The model under review builds one solid part; all positions refer to its coordinate system, in mm. A direction names the side the tool comes from. Give positions to 0.01 mm unless a question says otherwise; leave off trailing zeros. Write each loop counter-clockwise with the first axis right and the second up, starting at its lowest first coordinate (ties: lowest second). Pieces come first, ordered by that corner, then holes. Notation, with made-up numbers: (44.25, -10.5) - (67.25, -10.5) arc R28 ccw to (67.25, 7.5) - close; hole circle Ø3 at (35, 31.5). An arc over 180 degrees is marked (long way). One line per question, with ' | ' between items. Start each with the question number.
```python
from build123d import *

# Parameters (mm, degrees)
SKETCH1_W           = 80
SKETCH1_H           = 91
BOSS_EXTRUDE1_DEPTH = 10
SKETCH2_R           = 6.525
CUT_EXTRUDE1_DEPTH  = 76.543960712
SKETCH3_R           = 7.55
CUT_EXTRUDE2_DEPTH  = 1.1
CUT_EXTRUDE3_DEPTH  = 3
CIRPATTERN1_COUNT   = 3
SKETCH5_R           = 2.25
CUT_EXTRUDE4_DEPTH  = 76.543960712
SKETCH6_W           = 15
SKETCH6_H           = 60
CUT_EXTRUDE5_DEPTH  = 3.4
SKETCH7_R           = 1.75
CUT_EXTRUDE6_DEPTH  = 76.169475188


with BuildPart() as part:
    # Sketch1 → Boss-Extrude1 (new body)
    with BuildSketch(Plane.XY):
        with Locations((0, 17.8)):
            Rectangle(SKETCH1_W, SKETCH1_H)
    extrude(amount=BOSS_EXTRUDE1_DEPTH)

    # Sketch2 → Cut-Extrude1 (cut, through all)
    with BuildSketch(Plane.XY.offset(10)):
        Circle(SKETCH2_R)
    extrude(amount=-CUT_EXTRUDE1_DEPTH, mode=Mode.SUBTRACT)

    # Sketch3 → Cut-Extrude2 (cut)
    with BuildSketch(Plane.XY.offset(10)):
        Circle(SKETCH3_R)
    extrude(amount=-CUT_EXTRUDE2_DEPTH, mode=Mode.SUBTRACT)

    # Sketch4 → Cut-Extrude3 (cut)
    with BuildSketch(Plane.XY.offset(10)):
        with BuildLine():
            Line((-2, 35), (-2, 33))
            Line((-2, 33), (2, 33))
            Line((2, 33), (2, 35))
            ThreePointArc((2, 35), (3.9825, 36.9825), (5.965, 35))
            Line((5.965, 35), (5.965, 25))
            ThreePointArc((5.965, 25), (3.9825, 23.0175), (2, 25))
            Line((2, 25), (2, 27))
            Line((2, 27), (-2, 27))
            Line((-2, 27), (-2, 25))
            ThreePointArc((-2, 25), (-3.9825, 23.0175), (-5.965, 25))
            Line((-5.965, 25), (-5.965, 35))
            ThreePointArc((-5.965, 35), (-3.9825, 36.9825), (-2, 35))
        make_face()
    cut_extrude3 = extrude(amount=-CUT_EXTRUDE3_DEPTH, mode=Mode.SUBTRACT)

    # CirPattern1: Cut-Extrude3 ×3 about axis
    cirpattern1_axis = Axis((0, 0, 0), (0, 0, 1))
    for i in range(1, CIRPATTERN1_COUNT):
        add(cut_extrude3.rotate(cirpattern1_axis, i * 360 / CIRPATTERN1_COUNT), mode=Mode.SUBTRACT)

    # Sketch5 → Cut-Extrude4 (cut, through all)
    with BuildSketch(Plane.XY.offset(10)):
        with Locations((-19, 5.7)):
            Circle(SKETCH5_R)
        with Locations((19, 5.7)):
            Circle(SKETCH5_R)
        with Locations((0, 58.2)):
            Circle(SKETCH5_R)
    extrude(amount=-CUT_EXTRUDE4_DEPTH, mode=Mode.SUBTRACT)

    # Sketch6 → Cut-Extrude5 (cut)
    with BuildSketch(Plane.XY.offset(10)):
        with Locations((-32.5, 33.3)):
            Rectangle(SKETCH6_W, SKETCH6_H)
        with Locations((32.5, 33.3)):
            Rectangle(SKETCH6_W, SKETCH6_H)
    extrude(amount=-CUT_EXTRUDE5_DEPTH, mode=Mode.SUBTRACT)

    # Sketch7 → Cut-Extrude6 (cut, through all)
    with BuildSketch(Plane.XY.offset(6.6)):
        with Locations((-31, 21.075)):
            Circle(SKETCH7_R)
        with Locations((-31, 39.825)):
            Circle(SKETCH7_R)
        with Locations((31, 32.075)):
            Circle(SKETCH7_R)
        with Locations((31, 50.825)):
            Circle(SKETCH7_R)
    extrude(amount=-CUT_EXTRUDE6_DEPTH, mode=Mode.SUBTRACT)


solid = part.part
```
Item 1: For probe 1 along X at (y, z) = (26, 9.5) (3 decimals); probe 2 along Y at (x, z) = (0, 5) (3 decimals); probe 3 along Y at (x, z) = (-31, 1.5) (3 decimals), list the stretches that pass through material, from the lowest coordinate up.
Item 2: Take a section at D-D (z = 5.5). State how many separate pieces and enclosed holes the cut face has, plus the area to 3 significant figures.
Item 3: Take a section at A-A (y = 58.2). Give the boundary of the cut face in (x, z).
Item 4: Machinability: for faces 4 (the flat face through (-33, 34, 6.6)), 5 (the flat face through (32, 34, 6.6)), 6 (the cylindrical face through (-32.75, 39.9, 3.35)), 7 (the cylindrical face through (-30, -22, 9)), which of the approach directions +Z, -Z, +X, -X, +Y, -Y give a long, thin tool a straight path to every point of the face, cutting with its end or side? Answer none if there is none.
Item 5: Take a section at B-B (x = 0). Give the boundary of the cut face in (y, z) (3 decimals).
Item 6: The part is to be moulded in two halves that separate along X. For faces 1 (the flat face through (-40, 17, 4)), 2 (the flat face through (-1, -27.7, 5)), 3 (the flat face through (28.59, -16.48, 8.52)), say which applies: +X half, -X half, draft (parallel to the pull), parting line (faces both ways), or undercut.
Item 7: Take a section at C-C (y = 29). Give the boundary of the cut face in (x, z) (3 decimals).
Item 8: Clearance check with flat-ended pins moving along their axes: P1, Ø0.6, axis at y = 25.5, z = 8, coming from the +X side; P2, Ø16.5, axis at x = 36, y = 22, coming from the +Z side; P3, Ø2, axis at y = 34, z = 8.5, coming from the -X side. State where each tip first meets the part, or that it passes through.
Check sheet entries:
1) probe 1: x = -25 to -5.965, -2 to 2, 5.965 to 25 | probe 2: y = -27.7 to -6.525, 6.525 to 55.95, 60.45 to 63.3 | probe 3: y = -27.7 to 19.325, 22.825 to 38.075, 41.575 to 63.3
2) separate pieces: 1 | enclosed holes: 8 | area: 7,060 mm^2
3) outline: (-40, 0) - (-2.25, 0) - (-2.25, 10) - (-25, 10) - (-25, 6.6) - (-40, 6.6) - close; (2.25, 0) - (40, 0) - (40, 6.6) - (25, 6.6) - (25, 10) - (2.25, 10) - close
4) face 4: +Z, -X, +Y | face 5: +Z, +X, +Y | face 6: +Z, -Z | face 7: +Z
5) outline: (-27.7, 0) - (-6.525, 0) - (-6.525, 8.9) - (-7.55, 8.9) - (-7.55, 10) - (-27.7, 10) - close; (6.525, 0) - (55.95, 0) - (55.95, 10) - (33, 10) - (33, 7) - (27, 7) - (27, 10) - (7.55, 10) - (7.55, 8.9) - (6.525, 8.9) - close; (60.45, 0) - (63.3, 0) - (63.3, 10) - (60.45, 10) - close
6) face 1: -X half | face 2: draft | face 3: undercut
7) outline: (-40, 0) - (40, 0) - (40, 6.6) - (25, 6.6) - (25, 10) - (5.965, 10) - (5.965, 7) - (-5.965, 7) - (-5.965, 10) - (-25, 10) - (-25, 6.6) - (-40, 6.6) - close
8) P1: stops at x = 25 | P2: stops at z = 6.6 | P3: stops at x = -25
